Input: part model. Units: mm. Frame: model coordinates. A direction names the side the tool comes from. Give positions to 0.01 mm unless a question says otherwise; leave off trailing zeros. Write each loop counter-clockwise with the first axis right and the second up, starting at its lowest first coordinate (ties: lowest second). Pieces come first, ordered by that corner, then holes. Notation, with made-up numbers: (85, 10.5) - (120, 10.5) arc R20 cw to (120, 42.5) - close; hole circle Ø3 at (52, -40). An arc over 180 degrees is marked (long way). Use a Markdown table: item, result. Add a question column.
1. Section query D-D, the plane y = 13. Return loops of the section in (x, z).
2. Material intervals for probe 1 along Y at (x, z) = (10, 0.35); probe 2 along Y at (x, z) = (-3, -0.5); probe 3 along Y at (x, z) = (-10, 0.4), sorted ascending.
3. Section query C-C, the plane x = 10. Return loops of the section in (y, z), plus the area to 3 significant figures.
4. Set-up query: faces 1 (the flat face through (-7, 75, 3.065)), 2 (the flat face through (15, 118, 1)), 3 (the flat face through (13, 1, 8)). Return all of +Z, -Z, +X, -X, +Y, -Y with unobstructed straight access to the full face (end or side cutting, diameter ignored); none if empty.
5. Section query A-A, the plane x = -10. Return loops of the section in (y, z), plus the area to 3 significant figures.
6. Mould query, pull axis Y, two halves, no side actions, for faces 4 (the flat face through (0, 123, 1)), 5 (the flat face through (5, 2, 10)), 6 (the cylindrical face through (-8.925, 119.686, 1.029)). Classes: released by +Y, released by -Y, zero draft, split by the parting line, or undercut.
7. Section query B-B, the plane y = 118. Return loops of the section in (x, z), plus the area to 3 significant figures.
8. Pin query (flat end, axial travel): pin 1 (3.5 mm diameter, centred on y = 61.5, z = 2, fed in from +X); pin 2 (1.2 mm diameter, centred on y = 120, z = 1, fed in from +X); pin 3 (4.5 mm diameter, centred on x = 10, y = 118, fed in from +Z). Return the tip coordinate at first contact, or that it passes through.
```python
from build123d import *

# Parameters (mm, degrees)
EXTRUDE_1_DEPTH      = 3
SKETCH_4_W           = 15
SKETCH_4_H           = 10
EXTRUDE_3_DEPTH      = 3
SKETCH_5_W           = 10
SKETCH_5_H           = 4.129403984
EXTRUDE_4_DEPTH      = 120
EXTRUDE_4_DEPTH_BACK = 3
SKETCH_6_R           = 2
CUT_EXTRUDE_2_DEPTH  = 5.129403983
SKETCH_7_W           = 1.064701992
SKETCH_7_H           = 3
EXTRUDE_5_DEPTH      = 30
SKETCH_8_W           = 4.129403984
SKETCH_8_H           = 10
EXTRUDE_6_DEPTH      = 20
SKETCH_9_R           = 2
CUT_EXTRUDE_3_DEPTH  = 5.129403983


with BuildPart() as part:
    # 草图1 → 凸台-拉伸1 (new body)
    with BuildSketch(Plane(origin=(0, 0, 0), x_dir=(1, 0, 0), z_dir=(0, 1, 0))):
        with BuildLine():
            Line((25, 0), (0, 0))
            Line((0, 0), (0, -5))
            Line((0, -5), (2, -5))
            ThreePointArc((2, -5), (2.878679656, -2.878679656), (5, -2))
            Line((5, -2), (20, -2))
            ThreePointArc((20, -2), (22.121320344, -2.878679656), (23, -5))
            Line((23, -5), (25, -5))
            Line((25, -5), (25, 0))
        make_face()
        with BuildLine():
            Line((2, -5), (0, -5))
            Line((0, -5), (0, -10))
            Line((0, -10), (25, -10))
            Line((25, -10), (25, -5))
            Line((25, -5), (23, -5))
            ThreePointArc((23, -5), (22.121320344, -7.121320344), (20, -8))
            Line((20, -8), (5, -8))
            ThreePointArc((5, -8), (2.878679656, -7.121320344), (2, -5))
        make_face()
    extrude(amount=EXTRUDE_1_DEPTH)

    # 草图4 → 凸台-拉伸3 (add)
    with BuildSketch(Plane(origin=(0, 3, 0), x_dir=(1, 0, 0), z_dir=(0, 1, 0))):
        with Locations((-7.5, -5)):
            Rectangle(SKETCH_4_W, SKETCH_4_H)
    extrude(amount=-EXTRUDE_3_DEPTH)

    # 草图5 → 凸台-拉伸4 (add, two sides)
    with BuildSketch(Plane(origin=(0, 3, 0), x_dir=(1, 0, 0), z_dir=(0, 1, 0))) as extrude_4_sk:
        with Locations((-10, -1)):
            Rectangle(SKETCH_5_W, SKETCH_5_H)
    extrude(amount=EXTRUDE_4_DEPTH)
    extrude(extrude_4_sk.sketch, amount=-EXTRUDE_4_DEPTH_BACK)

    # 草图6 → 切除-拉伸2 (cut, through all)
    with BuildSketch(Plane.XY.offset(3.064701992)):
        with Locations((-10, 118)):
            Circle(SKETCH_6_R)
    extrude(amount=-CUT_EXTRUDE_2_DEPTH, mode=Mode.SUBTRACT)

    # 草图7 → 凸台-拉伸5 (add, through all)
    with BuildSketch(Plane(origin=(-5, 0, 0), x_dir=(0, 0, -1), z_dir=(1, 0, 0))):
        with Locations((0.532350996, 1.5)):
            Rectangle(SKETCH_7_W, SKETCH_7_H)
    extrude(amount=EXTRUDE_5_DEPTH)

    # 草图8 → 凸台-拉伸6 (add)
    with BuildSketch(Plane(origin=(-5, 0, 0), x_dir=(0, 0, -1), z_dir=(1, 0, 0))):
        with Locations((-1, 118)):
            Rectangle(SKETCH_8_W, SKETCH_8_H)
    extrude(amount=EXTRUDE_6_DEPTH)

    # 草图9 → 切除-拉伸3 (cut, through all)
    with BuildSketch(Plane.XY.offset(3.064701992)):
        with Locations((10, 118)):
            Circle(SKETCH_9_R)
    extrude(amount=-CUT_EXTRUDE_3_DEPTH, mode=Mode.SUBTRACT)


solid = part.part
```
Result sheet:
| question | item | result |
|---|---|---|
| 1 | outline | (-15, -1.06) - (-5, -1.06) - (-5, 3.06) - (-15, 3.06) - close |
| 2 | probe 1 | y = 0 to 3, 113 to 116, 120 to 123 |
| 2 | probe 2 | y = 0 to 3, 113 to 123 |
| 2 | probe 3 | y = 0 to 116, 120 to 123 |
| 3 | outline | (0, -1.06) - (3, -1.06) - (3, 2) - (0, 2) - close; (0, 8) - (3, 8) - (3, 10) - (0, 10) - close; (113, -1.06) - (116, -1.06) - (116, 3.06) - (113, 3.06) - close; (120, -1.06) - (123, -1.06) - (123, 3.06) - (120, 3.06) - close |
| 3 | area | 40.0 mm² |
| 4 | face 1 | +Z, +X, -X, +Y |
| 4 | face 2 | +Z, -Z, +X, +Y |
| 4 | face 3 | +Y, -Y |
| 5 | outline | (0, -1.06) - (116, -1.06) - (116, 3.06) - (3, 3.06) - (3, 10) - (0, 10) - close; (120, -1.06) - (123, -1.06) - (123, 3.06) - (120, 3.06) - close |
| 5 | area | 512 mm² |
| 6 | face 4 | released by +Y |
| 6 | face 5 | zero draft |
| 6 | face 6 | undercut |
| 7 | outline | (-15, -1.06) - (-12, -1.06) - (-12, 3.06) - (-15, 3.06) - close; (-8, -1.06) - (8, -1.06) - (8, 3.06) - (-8, 3.06) - close; (12, -1.06) - (15, -1.06) - (15, 3.06) - (12, 3.06) - close |
| 7 | area | 90.8 mm² |
| 8 | pin 1 | stops at x = -5 |
| 8 | pin 2 | stops at x = 15 |
| 8 | pin 3 | stops at z = 3.06 |
